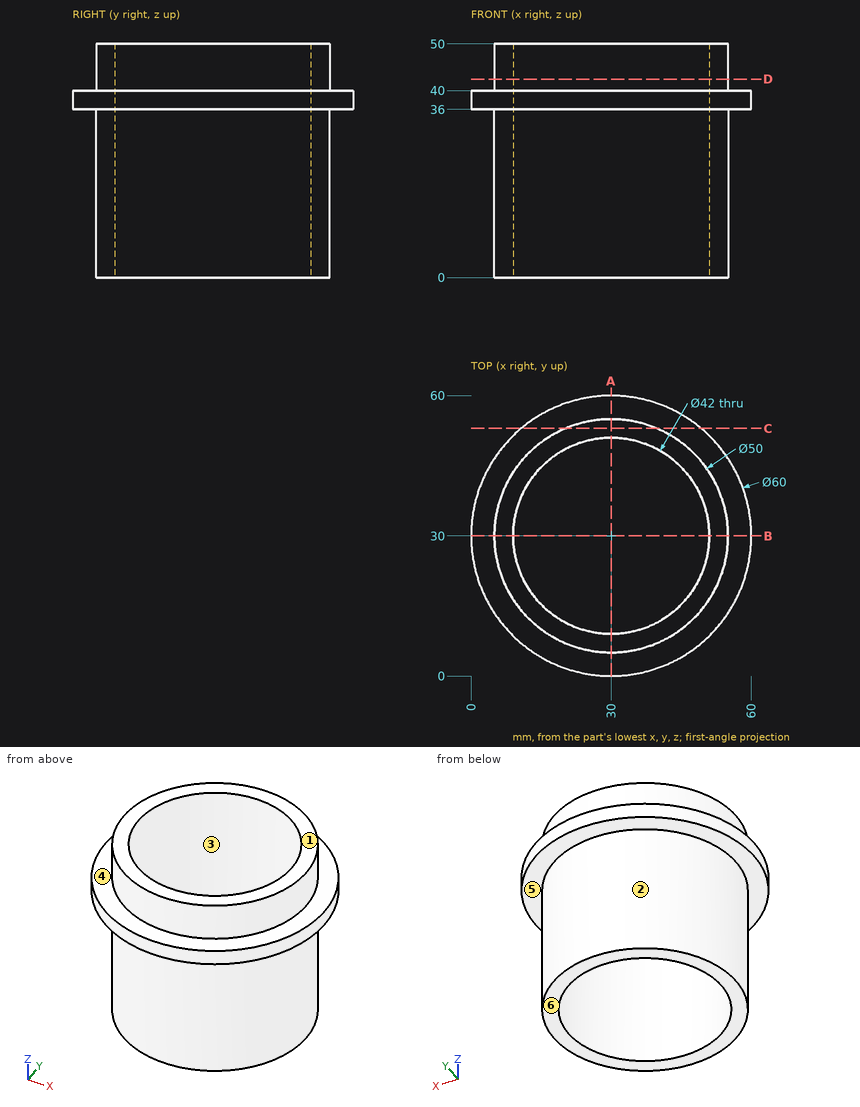
For this review, use the dimensioned drawing (mm, ordinates from the lowest corner) and the shaded views. A direction names the side the tool comes from. Give positions to 0.01 mm unless a question says otherwise; leave off trailing zeros. Write each loop counter-clockwise with the first axis right and the second up, starting at its lowest first coordinate (ties: lowest second). Pieces come first, ordered by that corner, then holes. Notation, with made-up numbers: M -22.5,59 L -10.5,59 A20 cw -10.5,72 Z; hole C 64.25,-13 d1. An arc over 180 degrees is marked long. Answer as a JSON object with one key per item and string values. Group by question number.
Item 1: Consider section A-A on x = 30. Write out the cut boundary in (y, z), plus the area to 3 significant figures.
Item 2: Consider section C-C on y = 53. Write out the cut boundary in (x, z).
Item 3: For probe 1 along X at (y, z) = (30, 27); probe 2 along X at (y, z) = (44.5, 10.5), list the stretches that pass through material, from the lowest coordinate up. Write a range as [from, to].
Item 4: For pin 1 Ø6 at (x, y) = (52.5, 8.5) entering from -Z; pin 2 Ø2 at (y, z) = (41, 42) entering from +X; pin 3 Ø6 at (x, z) = (34, 13.5) entering from -Y, all flat-tipped, find the tip position at first contact; note any pin that passes through.
Item 5: Consider section D-D on z = 42.5. Write out the cut boundary in (x, y).
Item 6: Draft analysis for pull direction Y (two halves, no side actions). For the marked faces 1, 2 and 3, state which applies: +Y half, -Y half, draft (parallel to the pull), parting line (faces both ways), or undercut.
Item 7: Tool access review of the marked faces 4, 5 and 6: name each direction out of +Z, -Z, +X, -X, +Y, -Y from which nothing blocks a thin tool from reaching the whole face with its end or side.
Check result:
{
 "1": {"outline": "M 0,36 L 5,36 L 5,0 L 9,0 L 9,50 L 5,50 L 5,40 L 0,40 Z; M 51,0 L 55,0 L 55,36 L 60,36 L 60,40 L 55,40 L 55,50 L 51,50 Z", "area": "440 mm^2"},
 "2": {"outline": "M 10.74,36 L 20.2,36 L 20.2,0 L 39.8,0 L 39.8,36 L 49.26,36 L 49.26,40 L 39.8,40 L 39.8,50 L 20.2,50 L 20.2,40 L 10.74,40 Z"},
 "3": {"probe 1": "x = [5, 9], [51, 55]", "probe 2": "x = [9.63, 14.81], [45.19, 50.37]"},
 "4": {"pin 1": "stops at z = 36", "pin 2": "stops at x = 52.91", "pin 3": "stops at y = 5.02"},
 "5": {"outline": "C 30,30 d50; hole C 30,30 d42"},
 "6": {"face 1": "draft", "face 2": "parting line", "face 3": "undercut"},
 "7": {"face 4": "+Z", "face 5": "-Z", "face 6": "-Z, +X, -X, +Y, -Y"}
}
